Check sheet for the modelled part. Datum: model origin and axes. Units: mm. Coordinates: 2 decimals unless noted, no trailing zeros. Order: outer loops, then holes, each group sorted by start corner. A loop starts at its lowest first (then second) coordinate and runs counter-clockwise, first axis right, second up.
Autodesk Fusion 360 part; units mm, degrees
sketch "スケッチ1" plane through (0, 0, 0) normal (0, 0, 1) x (1, 0, 0)
  line L0 (140, 0) -> (140, 216)
  line L1 (140, 216) -> (-140, 216)
  line L2 (-140, 216) -> (-140, 0)
  line L3 (-39, 132) -> (-35, 132)
  line L4 (-35, 132) -> (-35, 152)
  line L5 (-35, 152) -> (-39, 152)
  line L6 (-39, 152) -> (-39, 132)
  line L7 (35, 132) -> (39, 132)
  line L8 (39, 132) -> (39, 152)
  line L9 (39, 152) -> (35, 152)
  line L10 (35, 152) -> (35, 132)
  line L11 (-140, 0) -> (140, 0)
  line L12 (-35, 142) -> (-30, 142)
  line L13 (35, 142) -> (30, 142)
  line L14 (-130, 116) -> (-130, 206)
  line L15 (-130, 206) -> (130, 206)
  line L16 (130, 206) -> (130, 116)
  line L17 (15, 132) -> (-15, 132)
  line L18 (-15, 132) -> (-15, 102)
  line L19 (-15, 102) -> (15, 102)
  line L20 (15, 102) -> (15, 132)
  line L21 (15, 132) -> (-15, 102) construction
  line L22 (-15, 132) -> (15, 102) construction
  line L23 (-140, 82) -> (140, 82)
  line L24 (-80, 82) -> (-30, 82)
  line L25 (-30, 82) -> (-30, 86)
  line L26 (-30, 86) -> (-80, 86)
  line L27 (-80, 86) -> (-80, 82)
  line L28 (30, 82) -> (80, 82)
  line L29 (80, 82) -> (80, 86)
  line L30 (80, 86) -> (30, 86)
  line L31 (30, 86) -> (30, 82)
  line L32 (-130, 0) -> (-130, 25.5)
  line L33 (130, 0) -> (130, 25.5)
  line L34 (-50, 20) -> (50, 20)
  line L35 (50, 20) -> (50, 45)
  line L36 (50, 45) -> (-50, 45)
  line L37 (-50, 45) -> (-50, 20)
  line L38 (80, 20) -> (110, 20)
  line L39 (110, 20) -> (110, 45)
  line L40 (110, 45) -> (80, 45)
  line L41 (80, 45) -> (80, 20)
  line L42 (-80, 8) -> (-30, 8)
  line L43 (-30, 8) -> (-30, 12)
  line L44 (-30, 12) -> (-80, 12)
  line L45 (-80, 12) -> (-80, 8)
  line L46 (30, 8) -> (80, 8)
  line L47 (80, 8) -> (80, 12)
  line L48 (80, 12) -> (30, 12)
  line L49 (30, 12) -> (30, 8)
  line L50 (-80, 20) -> (-110, 20)
  line L51 (-110, 20) -> (-110, 45)
  line L52 (-110, 45) -> (-80, 45)
  line L53 (-80, 45) -> (-80, 20)
  line L54 (-130, 82) -> (-130, 99.5)
  line L55 (130, 82) -> (130, 99.5)
  point P0 (0, 216)
  point P1 (-100, 206)
  point P2 (100, 206)
  point P3 (0, 117)
  point P4 (0, 20)
  dimension "d3" = 4
  dimension "d5" = 20
  dimension "d10" = 216
  dimension "d20" = 280
  dimension "d24" = 5
  dimension "d25" = 5
  dimension "d26" = 10
  dimension "d27" = 10
  dimension "d28" = 10
  dimension "d29" = 90
  dimension "d30" = 100
  dimension "d31" = 100
  dimension "d45" = 30
  dimension "d46" = 30
  dimension "d51" = 20
  dimension "d52" = 50
  dimension "d53" = 50
  dimension "d54" = 4
  dimension "d57" = 10
  dimension "d58" = 10
  dimension "d59" = 25.5
  dimension "d60" = 25.5
  dimension "d63" = 25
  dimension "d67" = 8
  dimension "d68" = 30
  dimension "d69" = 30
  dimension "d70" = 50
  dimension "d71" = 50
  dimension "d72" = 4
  dimension "d73" = 20
  dimension "d74" = 100
  dimension "d75" = 30
  dimension "d76" = 30
  dimension "d77" = 70
  dimension "d78" = 17.5
  dimension "d79" = 50
  dimension "d80" = 35
  dimension "d81" = 35
  dimension "d82" = 30
  dimension "d83" = 30
extrude "押し出し1" add sketch "スケッチ1" along normal blind 4 contours L0 L2 L11 L23 L24 L28 | L0 L1 L2 L23 L25 L26 L27 L29 L30 L31
hole "穴1" at (-30, 142, 0) at (30, 142, 0) at (-130, 25.5, 0) at (130, 25.5, 0) at (130, 99.5, 0) at (-130, 99.5, 0) direction (0, 0, 1) diameter 3.2 depth 35 tip angle 118
hole "穴2" at (-130, 116, 0) at (-100, 206, 0) at (100, 206, 0) at (130, 116, 0) direction (0, 0, 1) diameter 4.3 depth 35 tip angle 118
fillet "フィレット1" radius 2 2 edges at (140, 216, 2) (-140, 216, 2)
equation "d59 = 13.5 mm + 12 mm"
equation "d60 = 13.5 mm + 12 mm"
(1) Cross-section at C-C (z = 3.1). Count the separate pieces of the cut face and the enclosed holes in it, and give its area (3 significant figures).
Filled in:
separate pieces: 1
enclosed holes: 20
area: 54,500 mm2
(2) Cross-section at B-B (x = 11). Enter the section's corners in (y, z).
Filled in:
outline: (0, 0) - (20, 0) - (20, 4) - (0, 4) - close; (45, 0) - (102, 0) - (102, 4) - (45, 4) - close; (132, 0) - (216, 0) - (216, 4) - (132, 4) - close
(3) Go/stop test with a flat-tipped pin: P1, Ø1.2, axis at x = -24, z = 2.5, coming from the -Y side. Record where the tip stops, or that it passes through.
Filled in:
P1: stops at y = 0
(4) Thickness scan on probe 1 along X at (y, z) = (133, 3.8); probe 2 along Y at (x, z) = (-45, 1.4); probe 3 along Y at (x, z) = (5.5, 1.5). Record the ranges inside material, lowest first.
Filled in:
probe 1: x = -140 to -39, -35 to 35, 39 to 140
probe 2: y = 0 to 8, 12 to 20, 45 to 82, 86 to 216
probe 3: y = 0 to 20, 45 to 102, 132 to 216
(5) Cross-section at A-A (x = -43). Enter the section's corners in (y, z).
Filled in:
outline: (0, 0) - (8, 0) - (8, 4) - (0, 4) - close; (12, 0) - (20, 0) - (20, 4) - (12, 4) - close; (45, 0) - (82, 0) - (82, 4) - (45, 4) - close; (86, 0) - (216, 0) - (216, 4) - (86, 4) - close
